```python
from build123d import *

# Parameters (mm, degrees)
F0_R      = 12.5
F1_DEPTH  = 10
F2_R      = 5
F3_DEPTH  = 10
F4_R      = 4.572682
F5_DEPTH  = 6
F6_R      = 1.5
F7_DEPTH  = 32
F8_R      = 2
F10_DEPTH = 4


with BuildPart() as f1:
    # F0 (on Top) → F1 (new body)
    with BuildSketch(Plane.XY):
        Circle(F0_R)
    extrude(amount=F1_DEPTH)

    # F2 (on face) → F3 (join)
    with BuildSketch(Plane.XY.offset(10)):
        Circle(F2_R)
    extrude(amount=F3_DEPTH)

    # F4 (on face) → F5 (join)
    with BuildSketch(Plane(origin=(0, 0, 0), x_dir=(1, 0, 0), z_dir=(0, 0, -1))):
        Circle(F4_R)
    extrude(amount=F5_DEPTH)

    # F6 (on face) → F7 (join)
    with BuildSketch(Plane(origin=(0, 0, -6), x_dir=(1, 0, 0), z_dir=(0, 0, -1))):
        Circle(F6_R)
    extrude(amount=F7_DEPTH)

    # F8
    f8_edges = [f1.edges().sort_by_distance(p)[0] for p in [
        (-12.5, 0, 0),
    ]]
    fillet(f8_edges, radius=F8_R)

    # F9 (on face) → F10 (cut)
    with BuildSketch(Plane(origin=(0, 0, -6), x_dir=(1, 0, 0), z_dir=(0, 0, -1))):
        with BuildLine():
            ThreePointArc((4.572682, 0), (4.055107, 2.113179), (2.61955, 3.747983))
            Line((2.61955, 3.747983), (2.61955, -3.747983))
            ThreePointArc((2.61955, -3.747983), (4.055107, -2.113179), (4.572682, 0))
        make_face()
        with BuildLine():
            Line((-2.61955, -3.747983), (-2.61955, 3.747983))
            ThreePointArc((-2.61955, 3.747983), (-4.572682, 0), (-2.61955, -3.747983))
        make_face()
    extrude(amount=-F10_DEPTH, mode=Mode.SUBTRACT)


solid = f1.part
```
Part model, mm, in its own coordinate system. A direction names the side the tool comes from. Round coordinates to 2 decimals unless told otherwise and drop trailing zeros. Write each loop counter-clockwise with the first axis right and the second up, starting at its lowest first coordinate (ties: lowest second). Pieces come first, ordered by that corner, then holes. Notation, with made-up numbers: (-2, 43.25) -> (57, 43.25) arc R18 cw to (57, 52.25) -> close; hole circle Ø4 at (41, -11). An arc over 180 degrees is marked (long way). Return JSON: item names as keys, results as strings. Group by question number.
Q1. Probe L1, parallel to Y at x = -4.25, z = 13.5; L2, parallel to Z at x = 3.25, y = -8.5; L3, parallel to Z at x = -3, y = -3.25. List the from-to ranges inside material, lowest first. Write a range as [from, to].
Q2. Pin check, flat tips, straight feed: pin 1 (10 mm diameter, centred on x = -6, y = 4.5, fed in from -Z); pin 2 (0.6 mm diameter, centred on x = -4, y = -1.5, fed in from -Z); pin 3 (4.5 mm diameter, centred on y = -1, z = -4.5, fed in from -X). Stop position of each tip, or through.
Q3. Saw through at A-A on x = 0. Write the cut outline in (y, z), plus the area to 3 significant figures.
Q4. Saw through at C-C on z = -11. Write the cut outline in (x, y), plus the area to 3 significant figures.
Q5. Which spindle directions (+Z, -Z, +X, -X, +Y, -Y) get a long thin tool onto all of the face, cutting with end or side? Do faces 1 (the flat face through (3, 0, -2)), 2 (the flat face through (-3, 0, -2)), 3 (the flat face through (5, -2, 0)), 4 (the flat face through (0, 0, -38)), 5 (the cylindrical face through (-1.08, -4.88, 14.93)). Say none if no direction does.
Q6. Saw through at B-B on y = 0. Write the cut outline in (x, z), plus the area to 3 significant figures.
Answer:
{
 "1": {"L1": "[-2.63, 2.63]", "L2": "[0, 10]", "L3": "[-2, 20]"},
 "2": {"pin 1": "z = -6", "pin 2": "z = -2", "pin 3": "x = -2.62"},
 "3": {"outline": "(-12.5, 2) arc R2 ccw to (-10.5, 0) -> (-4.57, 0) -> (-4.57, -6) -> (-1.5, -6) -> (-1.5, -38) -> (1.5, -38) -> (1.5, -6) -> (4.57, -6) -> (4.57, 0) -> (10.5, 0) arc R2 ccw to (12.5, 2) -> (12.5, 10) -> (5, 10) -> (5, 20) -> (-5, 20) -> (-5, 10) -> (-12.5, 10) -> close", "area": "499 mm2"},
 "4": {"outline": "circle Ø3 at (0, 0)", "area": "7.07 mm2"},
 "5": {"face 1": "-Z, +X, +Y, -Y", "face 2": "-Z, -X, +Y, -Y", "face 3": "-Z", "face 4": "-Z, +X, -X, +Y, -Y", "face 5": "+Z"},
 "6": {"outline": "(-12.5, 2) arc R2 ccw to (-10.5, 0) -> (-4.57, 0) -> (-4.57, -2) -> (-2.62, -2) -> (-2.62, -6) -> (-1.5, -6) -> (-1.5, -38) -> (1.5, -38) -> (1.5, -6) -> (2.62, -6) -> (2.62, -2) -> (4.57, -2) -> (4.57, 0) -> (10.5, 0) arc R2 ccw to (12.5, 2) -> (12.5, 10) -> (5, 10) -> (5, 20) -> (-5, 20) -> (-5, 10) -> (-12.5, 10) -> close", "area": "484 mm2"}
}
